from build123d import *

# Parameters (mm, degrees)
F0_R     = 12.7
F1_DEPTH = 2.54
F2_R     = 4.191
F3_DEPTH = 7.62
F4_R     = 3.302
F5_DEPTH = 7.621


with BuildPart() as f1:
    # F0 (on Top) → F1 (new body)
    with BuildSketch(Plane.XY):
        Circle(F0_R)
    extrude(amount=F1_DEPTH)

    # F2 (on Top) → F3 (join)
    with BuildSketch(Plane.XY):
        Circle(F2_R)
    extrude(amount=F3_DEPTH)

    # F4 (on Top) → F5 (cut, through all)
    with BuildSketch(Plane.XY):
        Circle(F4_R)
    extrude(amount=F5_DEPTH, mode=Mode.SUBTRACT)


solid = f1.part
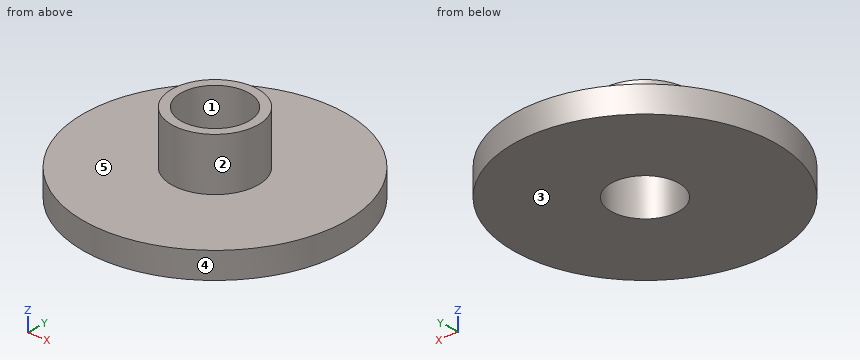
Check sheet for the modelled part. Datum: model origin and axes. Units: mm. Face numbers are marked on the shaded views. A direction names the side the tool comes from. Coordinates: 2 decimals unless noted, no trailing zeros. Write each loop counter-clockwise with the first axis right and the second up, starting at its lowest first coordinate (ties: lowest second). Pieces come first, ordered by that corner, then holes.
Item 1: Access from +Z, -Z, +X, -X, +Y, -Y to the whole of each face (thin tool, end or side, straight path). Record for the marked faces 4 and 5.
Numbers:
face 4: +Z, -Z
face 5: +Z
Item 2: Mould release check, pull along Y, two halves, no side actions. Record for the marked faces 1, 2 and 3: released by +Y, released by -Y, zero draft, split by the parting line, or undercut.
Numbers:
face 1: undercut
face 2: split by the parting line
face 3: zero draft
Item 3: Depth check by flat-ended pin: pin 1 Ø1 at (x, z) = (1, 3) entering from -Y; pin 2 Ø1.5 at (x, z) = (7, 1.5) entering from -Y; pin 3 Ø2 at (y, z) = (-8, 4.5) entering from -X; pin 4 Ø1 at (y, z) = (2, 4.5) entering from +X. Enter the tip coordinate at first touch or a pass-through.
Numbers:
pin 1: stops at y = -12.67
pin 2: stops at y = -11.06
pin 3: passes through
pin 4: stops at x = 3.91
Item 4: Cross-section at A-A on y = 0. Record the boundary of the cut face in (x, z), then the cut area to 3 significant figures.
Numbers:
outline: (-12.7, 0) - (-3.3, 0) - (-3.3, 7.62) - (-4.19, 7.62) - (-4.19, 2.54) - (-12.7, 2.54) - close; (3.3, 0) - (12.7, 0) - (12.7, 2.54) - (4.19, 2.54) - (4.19, 7.62) - (3.3, 7.62) - close
area: 56.8 mm2
Item 5: Scan lines: probe 1 along Y at (x, z) = (0, 2.5); probe 2 along Y at (x, z) = (0, 5.25). Record each from-to range of solid material in increasing order.
Numbers:
probe 1: y = -12.7 to -3.3, 3.3 to 12.7
probe 2: y = -4.19 to -3.3, 3.3 to 4.19
Item 6: Cross-section at D-D on y = -8.25. Record the boundary of the cut face in (x, z), then the cut area to 3 significant figures.
Numbers:
outline: (-9.66, 0) - (9.66, 0) - (9.66, 2.54) - (-9.66, 2.54) - close
area: 49.0 mm2
Item 7: Cross-section at C-C on z = 3.25. Record the boundary of the cut face in (x, y).
Numbers:
outline: circle Ø8.38 at (0, 0); hole circle Ø6.6 at (0, 0)
